Verification items for the finished model (mm, model axes). Give positions to 0.01 mm unless a question says otherwise; leave off trailing zeros. Answer as a JSON object with one key per item and string values.
```python
from build123d import *

# Parameters (mm, degrees)
SKETCH4_R           = 169.4688
SKETCH4_R_2         = 3.2385
BOSS_EXTRUDE2_DEPTH = 0.75
SKETCH8_R           = 3.5
CUT_EXTRUDE2_DEPTH  = 1.7500001


with BuildPart() as part:
    # Sketch4 → Boss-Extrude2 (new body)
    with BuildSketch(Plane.XY):
        with BuildLine():
            Line((-7.735342369, 190.342886598), (7.735342369, 190.342886598))
            add(Edge.make_bspline(
                [(7.735342369, 190.342886598), (43.849986057, 163.650375876), (88.472440301, 168.709446408)],
                knots=[0, 0, 0, 1, 1, 1], degree=2))
            Line((88.472440301, 168.709446408), (101.870446297, 160.974104039))
            add(Edge.make_bspline(
                [(101.870446297, 160.974104039), (119.800389819, 119.800389819), (160.974104039, 101.870446297)],
                knots=[0, 0, 0, 1, 1, 1], degree=2))
            Line((160.974104039, 101.870446297), (168.709446408, 88.472440301))
            add(Edge.make_bspline(
                [(168.709446408, 88.472440301), (163.650375876, 43.849986057), (190.342886598, 7.735342369)],
                knots=[0, 0, 0, 1, 1, 1], degree=2))
            Line((190.342886598, 7.735342369), (190.342886598, -7.735342369))
            add(Edge.make_bspline(
                [(190.342886598, -7.735342369), (163.650375876, -43.849986057), (168.709446408, -88.472440301)],
                knots=[0, 0, 0, 1, 1, 1], degree=2))
            Line((168.709446408, -88.472440301), (160.974104039, -101.870446297))
            add(Edge.make_bspline(
                [(160.974104039, -101.870446297), (119.800389819, -119.800389819), (101.870446297, -160.974104039)],
                knots=[0, 0, 0, 1, 1, 1], degree=2))
            Line((101.870446297, -160.974104039), (88.472440301, -168.709446408))
            add(Edge.make_bspline(
                [(88.472440301, -168.709446408), (43.849986057, -163.650375876), (7.735342369, -190.342886598)],
                knots=[0, 0, 0, 1, 1, 1], degree=2))
            Line((7.735342369, -190.342886598), (-7.735342369, -190.342886598))
            add(Edge.make_bspline(
                [(-7.735342369, -190.342886598), (-43.849986057, -163.650375876), (-88.472440301, -168.709446408)],
                knots=[0, 0, 0, 1, 1, 1], degree=2))
            Line((-88.472440301, -168.709446408), (-101.870446297, -160.974104039))
            add(Edge.make_bspline(
                [(-101.870446297, -160.974104039), (-119.800389819, -119.800389819), (-160.974104039, -101.870446297)],
                knots=[0, 0, 0, 1, 1, 1], degree=2))
            Line((-160.974104039, -101.870446297), (-168.709446408, -88.472440301))
            add(Edge.make_bspline(
                [(-168.709446408, -88.472440301), (-163.650375876, -43.849986057), (-190.342886598, -7.735342369)],
                knots=[0, 0, 0, 1, 1, 1], degree=2))
            Line((-190.342886598, -7.735342369), (-190.342886598, 7.735342369))
            add(Edge.make_bspline(
                [(-190.342886598, 7.735342369), (-163.877360858, 32.597233808), (-178.814084455, 65.694544678)],
                knots=[0, 0, 0, 1, 1, 1], degree=2))
            Line((-178.814084455, 65.694544678), (-172.893709719, 79.987593661))
            add(Edge.make_bspline(
                [(-172.893709719, 79.987593661), (-138.92851822, 92.829068072), (-140.062458908, 129.12303282)],
                knots=[0, 0, 0, 1, 1, 1], degree=2))
            Line((-140.062458908, 129.12303282), (-129.12303282, 140.062458908))
            add(Edge.make_bspline(
                [(-129.12303282, 140.062458908), (-92.829068072, 138.92851822), (-79.987593661, 172.893709719)],
                knots=[0, 0, 0, 1, 1, 1], degree=2))
            Line((-79.987593661, 172.893709719), (-65.694544678, 178.814084455))
            add(Edge.make_bspline(
                [(-65.694544678, 178.814084455), (-32.597233808, 163.877360858), (-7.735342369, 190.342886598)],
                knots=[0, 0, 0, 1, 1, 1], degree=2))
        make_face()
        Circle(SKETCH4_R, mode=Mode.SUBTRACT)
        with Locations((0, 184.785)):
            Circle(SKETCH4_R_2, mode=Mode.SUBTRACT)
        with Locations((-160.028504238, -92.3925)):
            Circle(SKETCH4_R_2, mode=Mode.SUBTRACT)
        with Locations((-92.3925, -160.028504238)):
            Circle(SKETCH4_R_2, mode=Mode.SUBTRACT)
        with Locations((0, -184.785)):
            Circle(SKETCH4_R_2, mode=Mode.SUBTRACT)
        with Locations((92.3925, -160.028504238)):
            Circle(SKETCH4_R_2, mode=Mode.SUBTRACT)
        with Locations((160.028504238, -92.3925)):
            Circle(SKETCH4_R_2, mode=Mode.SUBTRACT)
        with Locations((184.785, 0)):
            Circle(SKETCH4_R_2, mode=Mode.SUBTRACT)
        with Locations((160.028504238, 92.3925)):
            Circle(SKETCH4_R_2, mode=Mode.SUBTRACT)
        with Locations((92.3925, 160.028504238)):
            Circle(SKETCH4_R_2, mode=Mode.SUBTRACT)
        with Locations((-70.71415805, 170.719079415)):
            Circle(SKETCH4_R_2, mode=Mode.SUBTRACT)
        with Locations((-130.662726562, 130.662726562)):
            Circle(SKETCH4_R_2, mode=Mode.SUBTRACT)
        with Locations((-170.719079415, 70.71415805)):
            Circle(SKETCH4_R_2, mode=Mode.SUBTRACT)
        with Locations((-184.785, 0)):
            Circle(SKETCH4_R_2, mode=Mode.SUBTRACT)
    extrude(amount=BOSS_EXTRUDE2_DEPTH)

    # Sketch8 → Cut-Extrude2 (cut, through all)
    with BuildSketch(Plane.XY.offset(0.75)):
        with Locations((14.2615, 179.5235)):
            Circle(SKETCH8_R)
        with Locations((-176.455298363, 13.2615)):
            Circle(SKETCH8_R)
        with Locations((102.112571296, 148.341161576)):
            Circle(SKETCH8_R)
        with Locations((162.602661576, 77.410928704)):
            Circle(SKETCH8_R)
        with Locations((179.5235, -14.2615)):
            Circle(SKETCH8_R)
        with Locations((148.341161576, -102.112571296)):
            Circle(SKETCH8_R)
        with Locations((77.410928704, -162.602661576)):
            Circle(SKETCH8_R)
        with Locations((-14.2615, -179.5235)):
            Circle(SKETCH8_R)
        with Locations((-102.112571296, -148.341161576)):
            Circle(SKETCH8_R)
        with Locations((-162.602661576, -77.410928704)):
            Circle(SKETCH8_R)
        with Locations((-157.948482222, 79.778547657)):
            Circle(SKETCH8_R)
        with Locations((-115.39544147, 134.150034627)):
            Circle(SKETCH8_R)
        with Locations((-55.274490816, 168.098394899)):
            Circle(SKETCH8_R)
    extrude(amount=-CUT_EXTRUDE2_DEPTH, mode=Mode.SUBTRACT)


solid = part.part
```
1) Go/stop test with flat-tipped pins: pin 1 (5.5 mm diameter, centred on x = 179.52, y = -14.26, fed in from -Z); pin 2 (8 mm diameter, centred on x = 77.41, y = -162.6, fed in from +Z). Record where each tip stops, or that it passes through.
Completed:
{"pin 1": "passes through", "pin 2": "stops at z = 0.75"}
2) Release check for a two-part mould opening along Y. For faces 1 (the face through (-36.74, -165.44, 0.37)), 2 (the face through (-134.669, 134.516, 0.37)), 3 (the face through (170, 1, 0)) record: pulls with the +Y half, pulls with the -Y half, needs draft (parallel to the pull), parting line crosses it, or undercut.
Completed:
{"face 1": "undercut", "face 2": "pulls with the +Y half", "face 3": "needs draft"}
3) Section check A-A on z = 0.45. Count the separate pieces of the cut face and the enclosed holes in it, and give its area (3 significant figures).
Completed:
{"separate pieces": "1", "enclosed holes": "27", "area": "14,400 mm2"}
4) Thickness scan on L1, parallel to X at y = -33, z = 0.6; L2, parallel to Y at x = 93.5, z = 0.15; L3, parallel to X at y = -106, z = 0.3. Record the ranges inside material, lowest first.
Completed:
{"L1": "x = -175.98 to -166.22, 166.22 to 175.98", "L2": "y = -165.81 to -163.07, -156.99 to -141.34, 141.34 to 156.99, 163.07 to 165.81", "L3": "x = -152.38 to -132.23, 132.23 to 152.38"}
